Design review of the part built by this model. Coordinates are the model's own, in mm. Coordinates: 2 decimals unless noted, no trailing zeros. Use a Markdown table: item, result. Add a question column.
Q1. Clearance check with flat-ended pins moving along their axes: pin 1 Ø0.6 at (y, z) = (14.5, 428.5) entering from +X; pin 2 Ø2 at (x, y) = (0.5, -1) entering from +Z; pin 3 Ø0.6 at (x, z) = (13.5, 213.5) entering from -Y; pin 4 Ø4 at (y, z) = (0, 90) entering from +X. State where each tip first meets the part, or that it passes through.
Q2. Take a section at A-A on z = 493.5. Count the separate pieces of the cut face and the enclosed holes in it, plus the area to 3 significant figures.
Q3. For probe 1 along X at (y, z) = (13.75, 642); probe 2 along Y at (x, z) = (6.5, 79); probe 3 along X at (y, z) = (11.5, 38), list the stretches that pass through material, from the lowest coordinate up.
from build123d import *

# Parameters (mm, degrees)
CROQUIS1_R              = 1.25
CROQUIS1_R_2            = 3.4
SALIENTE_EXTRUIR1_DEPTH = 675


with BuildPart() as part:
    # Croquis1 → Saliente-Extruir1 (new body)
    with BuildSketch(Plane.XY):
        with BuildLine():
            Line((-4.161522369, 5.8), (4.161522369, 5.8))
            ThreePointArc((4.161522369, 5.8), (4.238059055, 5.815224093), (4.302943725, 5.858578644))
            Line((4.302943725, 5.858578644), (8.191421356, 9.747056275))
            ThreePointArc((8.191421356, 9.747056275), (8.234775907, 9.811940945), (8.25, 9.888477631))
            Line((8.25, 9.888477631), (8.25, 12.6))
            ThreePointArc((8.25, 12.6), (8.191421356, 12.741421356), (8.05, 12.8))
            Line((8.05, 12.8), (4.3, 12.8))
            ThreePointArc((4.3, 12.8), (4.158578644, 12.858578644), (4.1, 13))
            Line((4.1, 13), (4.1, 13.7))
            ThreePointArc((4.1, 13.7), (4.158578644, 13.841421356), (4.3, 13.9))
            Line((4.3, 13.9), (4.9, 13.9))
            ThreePointArc((4.9, 13.9), (5.041421356, 13.958578644), (5.1, 14.1))
            Line((5.1, 14.1), (5.1, 14.8))
            ThreePointArc((5.1, 14.8), (5.158578644, 14.941421356), (5.3, 15))
            Line((5.3, 15), (12.8, 15))
            ThreePointArc((12.8, 15), (14.355634919, 14.355634919), (15, 12.8))
            Line((15, 12.8), (15, 5.3))
            ThreePointArc((15, 5.3), (14.941421356, 5.158578644), (14.8, 5.1))
            Line((14.8, 5.1), (13.9, 5.1))
            Line((13.9, 5.1), (13.9, 4.3))
            ThreePointArc((13.9, 4.3), (13.841421356, 4.158578644), (13.7, 4.1))
            Line((13.7, 4.1), (13, 4.1))
            ThreePointArc((13, 4.1), (12.858578644, 4.158578644), (12.8, 4.3))
            Line((12.8, 4.3), (12.8, 8.05))
            ThreePointArc((12.8, 8.05), (12.741421356, 8.191421356), (12.6, 8.25))
            Line((12.6, 8.25), (9.888477631, 8.25))
            ThreePointArc((9.888477631, 8.25), (9.811940945, 8.234775907), (9.747056275, 8.191421356))
            Line((9.747056275, 8.191421356), (5.858578644, 4.302943725))
            ThreePointArc((5.858578644, 4.302943725), (5.815224093, 4.238059055), (5.8, 4.161522369))
            Line((5.8, 4.161522369), (5.8, -4.161522369))
            ThreePointArc((5.8, -4.161522369), (5.815224093, -4.238059055), (5.858578644, -4.302943725))
            Line((5.858578644, -4.302943725), (9.747056275, -8.191421356))
            ThreePointArc((9.747056275, -8.191421356), (9.811940945, -8.234775907), (9.888477631, -8.25))
            Line((9.888477631, -8.25), (12.6, -8.25))
            ThreePointArc((12.6, -8.25), (12.741421356, -8.191421356), (12.8, -8.05))
            Line((12.8, -8.05), (12.8, -4.3))
            ThreePointArc((12.8, -4.3), (12.858578644, -4.158578644), (13, -4.1))
            Line((13, -4.1), (13.7, -4.1))
            ThreePointArc((13.7, -4.1), (13.841421356, -4.158578644), (13.9, -4.3))
            Line((13.9, -4.3), (13.9, -5.1))
            Line((13.9, -5.1), (14.8, -5.1))
            ThreePointArc((14.8, -5.1), (14.941421356, -5.158578644), (15, -5.3))
            Line((15, -5.3), (15, -12.8))
            ThreePointArc((15, -12.8), (14.355634919, -14.355634919), (12.8, -15))
            Line((12.8, -15), (5.3, -15))
            ThreePointArc((5.3, -15), (5.158578644, -14.941421356), (5.1, -14.8))
            Line((5.1, -14.8), (5.1, -14.1))
            ThreePointArc((5.1, -14.1), (5.041421356, -13.958578644), (4.9, -13.9))
            Line((4.9, -13.9), (4.3, -13.9))
            ThreePointArc((4.3, -13.9), (4.158578644, -13.841421356), (4.1, -13.7))
            Line((4.1, -13.7), (4.1, -13))
            ThreePointArc((4.1, -13), (4.158578644, -12.858578644), (4.3, -12.8))
            Line((4.3, -12.8), (8.05, -12.8))
            ThreePointArc((8.05, -12.8), (8.191421356, -12.741421356), (8.25, -12.6))
            Line((8.25, -12.6), (8.25, -9.888477631))
            ThreePointArc((8.25, -9.888477631), (8.234775907, -9.811940945), (8.191421356, -9.747056275))
            Line((8.191421356, -9.747056275), (4.302943725, -5.858578644))
            ThreePointArc((4.302943725, -5.858578644), (4.238059055, -5.815224093), (4.161522369, -5.8))
            Line((4.161522369, -5.8), (-4.161522369, -5.8))
            ThreePointArc((-4.161522369, -5.8), (-4.238059055, -5.815224093), (-4.302943725, -5.858578644))
            Line((-4.302943725, -5.858578644), (-8.191421356, -9.747056275))
            ThreePointArc((-8.191421356, -9.747056275), (-8.234775907, -9.811940945), (-8.25, -9.888477631))
            Line((-8.25, -9.888477631), (-8.25, -12.6))
            ThreePointArc((-8.25, -12.6), (-8.191421356, -12.741421356), (-8.05, -12.8))
            Line((-8.05, -12.8), (-4.3, -12.8))
            ThreePointArc((-4.3, -12.8), (-4.158578644, -12.858578644), (-4.1, -13))
            Line((-4.1, -13), (-4.1, -13.7))
            ThreePointArc((-4.1, -13.7), (-4.158578644, -13.841421356), (-4.3, -13.9))
            Line((-4.3, -13.9), (-4.9, -13.9))
            ThreePointArc((-4.9, -13.9), (-5.041421356, -13.958578644), (-5.1, -14.1))
            Line((-5.1, -14.1), (-5.1, -14.8))
            ThreePointArc((-5.1, -14.8), (-5.158578644, -14.941421356), (-5.3, -15))
            Line((-5.3, -15), (-12.8, -15))
            ThreePointArc((-12.8, -15), (-14.355634919, -14.355634919), (-15, -12.8))
            Line((-15, -12.8), (-15, -5.3))
            ThreePointArc((-15, -5.3), (-14.941421356, -5.158578644), (-14.8, -5.1))
            Line((-14.8, -5.1), (-13.9, -5.1))
            Line((-13.9, -5.1), (-13.9, -4.3))
            ThreePointArc((-13.9, -4.3), (-13.841421356, -4.158578644), (-13.7, -4.1))
            Line((-13.7, -4.1), (-13, -4.1))
            ThreePointArc((-13, -4.1), (-12.858578644, -4.158578644), (-12.8, -4.3))
            Line((-12.8, -4.3), (-12.8, -8.05))
            ThreePointArc((-12.8, -8.05), (-12.741421356, -8.191421356), (-12.6, -8.25))
            Line((-12.6, -8.25), (-9.888477631, -8.25))
            ThreePointArc((-9.888477631, -8.25), (-9.811940945, -8.234775907), (-9.747056275, -8.191421356))
            Line((-9.747056275, -8.191421356), (-5.858578644, -4.302943725))
            ThreePointArc((-5.858578644, -4.302943725), (-5.815224093, -4.238059055), (-5.8, -4.161522369))
            Line((-5.8, -4.161522369), (-5.8, 4.161522369))
            ThreePointArc((-5.8, 4.161522369), (-5.815224093, 4.238059055), (-5.858578644, 4.302943725))
            Line((-5.858578644, 4.302943725), (-9.747056275, 8.191421356))
            ThreePointArc((-9.747056275, 8.191421356), (-9.811940945, 8.234775907), (-9.888477631, 8.25))
            Line((-9.888477631, 8.25), (-12.6, 8.25))
            ThreePointArc((-12.6, 8.25), (-12.741421356, 8.191421356), (-12.8, 8.05))
            Line((-12.8, 8.05), (-12.8, 4.3))
            ThreePointArc((-12.8, 4.3), (-12.858578644, 4.158578644), (-13, 4.1))
            Line((-13, 4.1), (-13.7, 4.1))
            ThreePointArc((-13.7, 4.1), (-13.841421356, 4.158578644), (-13.9, 4.3))
            Line((-13.9, 4.3), (-13.9, 5.1))
            Line((-13.9, 5.1), (-14.8, 5.1))
            ThreePointArc((-14.8, 5.1), (-14.941421356, 5.158578644), (-15, 5.3))
            Line((-15, 5.3), (-15, 12.8))
            ThreePointArc((-15, 12.8), (-14.355634919, 14.355634919), (-12.8, 15))
            Line((-12.8, 15), (-5.3, 15))
            ThreePointArc((-5.3, 15), (-5.158578644, 14.941421356), (-5.1, 14.8))
            Line((-5.1, 14.8), (-5.1, 14.1))
            ThreePointArc((-5.1, 14.1), (-5.041421356, 13.958578644), (-4.9, 13.9))
            Line((-4.9, 13.9), (-4.3, 13.9))
            ThreePointArc((-4.3, 13.9), (-4.158578644, 13.841421356), (-4.1, 13.7))
            Line((-4.1, 13.7), (-4.1, 13))
            ThreePointArc((-4.1, 13), (-4.158578644, 12.858578644), (-4.3, 12.8))
            Line((-4.3, 12.8), (-8.05, 12.8))
            ThreePointArc((-8.05, 12.8), (-8.191421356, 12.741421356), (-8.25, 12.6))
            Line((-8.25, 12.6), (-8.25, 9.888477631))
            ThreePointArc((-8.25, 9.888477631), (-8.234775907, 9.811940945), (-8.191421356, 9.747056275))
            Line((-8.191421356, 9.747056275), (-4.302943725, 5.858578644))
            ThreePointArc((-4.302943725, 5.858578644), (-4.238059055, 5.815224093), (-4.161522369, 5.8))
        make_face()
        with Locations((11.625, 11.625)):
            Circle(CROQUIS1_R, mode=Mode.SUBTRACT)
        with Locations((11.625, -11.625)):
            Circle(CROQUIS1_R, mode=Mode.SUBTRACT)
        with Locations((-11.625, -11.625)):
            Circle(CROQUIS1_R, mode=Mode.SUBTRACT)
        with Locations((-11.625, 11.625)):
            Circle(CROQUIS1_R, mode=Mode.SUBTRACT)
        Circle(CROQUIS1_R_2, mode=Mode.SUBTRACT)
    extrude(amount=SALIENTE_EXTRUIR1_DEPTH)


solid = part.part
Answer list:
| question | item | result |
|---|---|---|
| 1 | pin 1 | x = 14.5 |
| 1 | pin 2 | through |
| 1 | pin 3 | y = -14.96 |
| 1 | pin 4 | x = 5.8 |
| 2 | separate pieces | 1 |
| 2 | enclosed holes | 5 |
| 2 | area | 361 mm² |
| 3 | probe 1 | -14.78 to -4.11, 4.11 to 14.78 |
| 3 | probe 2 | -15 to -12.8, -8.06 to -4.94, 4.94 to 8.06, 12.8 to 15 |
| 3 | probe 3 | -15 to -12.87, -10.38 to -8.25, 8.25 to 10.38, 12.87 to 15 |
